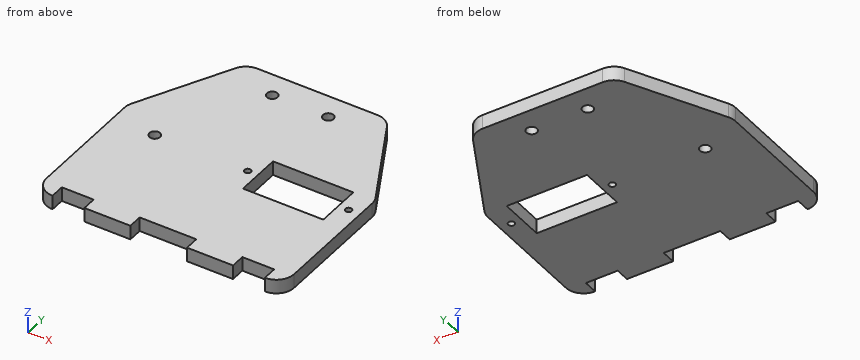
Solid Edge part; units mm, degrees
sketch "Sketch1" plane through (39.9722, 24.5714, 4) normal (0, 0, 1) x (1, 0, 0)
  line L0 (-35, 5.5) -> (-35, -34.5)
  line L1 (-35, -34.5) -> (-30, -34.5)
  line L2 (-30, -34.5) -> (-30, -30.5)
  line L3 (-30, -30.5) -> (-21, -30.5)
  line L4 (-21, -30.5) -> (-21, -34.5)
  line L5 (-21, -34.5) -> (-8, -34.5)
  line L6 (-8, -34.5) -> (-8, -30.5)
  line L7 (-8, -30.5) -> (8, -30.5)
  line L8 (8, -30.5) -> (8, -34.5)
  line L9 (8, -34.5) -> (21, -34.5)
  line L10 (21, -34.5) -> (21, -30.5)
  line L11 (21, -30.5) -> (30, -30.5)
  line L12 (30, -30.5) -> (30, -34.5)
  line L13 (30, -34.5) -> (35, -34.5)
  line L14 (35, -34.5) -> (35, 5.5)
  line L15 (35, 5.5) -> (19.7554, 34.5)
  line L16 (19.7554, 34.5) -> (-20.2446, 34.5)
  line L17 (-20.2446, 34.5) -> (-35, 5.5)
  line L18 (28, 5.5) -> (28.86, 5.5)
  line L19 (28.86, 5.5) -> (28.86, -7.5)
  line L20 (28, -7.5) -> (28.86, -7.5)
  line L21 (6.8, -7.5) -> (28, -7.5)
  line L22 (6.16, -7.5) -> (6.8, -7.5)
  line L23 (6.16, 5.5) -> (6.16, -7.5)
  line L24 (6.8, 5.5) -> (6.16, 5.5)
  line L25 (6.8, 5.5) -> (28, 5.5)
extrude "Protrusion1" add sketch "Sketch1" along normal blind 4
hole "Furo_18" at (43.2322, 23.5714, 8) direction (0, 0, -1) diameter 1.8 end up to next
hole "Hole1" at (71.7322, 23.5714, 8) direction (0, 0, -1) diameter 1.8 end up to next
hole "Furo_23" at (31.554, 52.0714, 8) direction (0, 0, -1) diameter 3 end up to next
hole "Hole2" at (47.394, 52.0714, 8) direction (0, 0, -1) diameter 3 end up to next
hole "Hole3" at (16.9722, 23.5714, 8) direction (0, 0, -1) diameter 3 end up to next
fillet "Redondo_6" radius 5 4 edges at (59.7276, 59.0714, 6) (74.9722, 30.0714, 6) (19.7276, 59.0714, 6) (4.9722, 30.0714, 6)
fillet "Redondo_7" radius 5 2 edges at (4.9722, -9.9286, 6) (74.9722, -9.9286, 6)
Source: CAD feature listing. Evaluate the final solid. Frame: model axes, mm. Coordinates: 2 decimals unless noted, no trailing zeros. Order: outer loops, then holes, each group sorted by start corner. A loop starts at its lowest first (then second) coordinate and runs counter-clockwise, first axis right, second up.
Item 1: Cut plane D-D (y = 49). Return loops of the section in (x, z).
Output values:
outline: (14.6, 4) - (65.02, 4) - (65.02, 8) - (14.6, 8) - close
Item 2: Cut plane C-C (x = 41). Return loops of the section in (y, z), plus the area to 3 significant figures.
Output values:
outline: (-5.93, 4) - (59.07, 4) - (59.07, 8) - (-5.93, 8) - close
area: 260 mm2
Item 3: Cut plane A-A (x = 65). Return loops of the section in (y, z), plus the area to 3 significant figures.
Output values:
outline: (-5.93, 4) - (17.07, 4) - (17.07, 8) - (-5.93, 8) - close; (30.07, 4) - (49.04, 4) - (49.04, 8) - (30.07, 8) - close
area: 168 mm2
Item 4: Material intervals for line 1 (Y direction, x = 54, z = 5.7); line 2 (X direction, y = 24, z = 6.1); line 3 (X direction, y = 22, z = 6.9), sorted ascending.
Output values:
line 1: y = -9.93 to 17.07, 30.07 to 59.07
line 2: x = 4.97 to 15.53, 18.41 to 42.44, 44.02 to 46.13, 68.83 to 70.94, 72.52 to 74.97
line 3: x = 4.97 to 46.13, 68.83 to 74.97
Item 5: First-contact query: P1, Ø2.5, axis at x = 31.55, y = 52.07, coming from the +Z side; P2, Ø8, axis at x = 65, y = 21.5, coming from the -Z side; P3, Ø2, axis at x = 14.5, z = 6.5, coming from the -Y side; P4, Ø1.2, axis at y = -7.5, z = 5.5, coming from the -X side. Flat tips, straight axial feed; report the tip coordinate or a pass-through.
Output values:
P1: passes through
P2: stops at z = 4
P3: stops at y = -5.93
P4: stops at x = 5.38
Item 6: Cut plane B-B (z = 5.3). Count the separate pieces of the cut face and the enclosed holes in it, plus the area to 3 significant figures.
Output values:
separate pieces: 1
enclosed holes: 6
area: 3,920 mm2
